```python
from build123d import *

# Parameters (mm, degrees)
SKETCH1_W               = 35
SKETCH1_H               = 17
BOSS_EXTRUDE1_DEPTH     = 0.5
SKETCH2_W               = 4.5
SKETCH2_H               = 8
BOSS_EXTRUDE2_DEPTH     = 3
SKETCH3_W               = 10.6
SKETCH3_H               = 15.6
BOSS_EXTRUDE3_DEPTH     = 1.5
CUT_EXTRUDE1_DEPTH      = 20.685019685
CUT_EXTRUDE1_DEPTH_BACK = 20.685019685
SKETCH4_R               = 1.1


with BuildPart() as part:
    # Sketch1 → Boss-Extrude1 (new, symmetric)
    with BuildSketch(Plane(origin=(0, 0, 0), x_dir=(1, 0, 0), z_dir=(0, 1, 0))):
        Rectangle(SKETCH1_W, SKETCH1_H)
    extrude(amount=BOSS_EXTRUDE1_DEPTH, both=True)

    # Sketch2 → Boss-Extrude2 (add)
    with BuildSketch(Plane(origin=(0, 0.5, 0), x_dir=(1, 0, 0), z_dir=(0, 1, 0))):
        with Locations((-15.25, -2.8)):
            Rectangle(SKETCH2_W, SKETCH2_H)
    extrude(amount=BOSS_EXTRUDE2_DEPTH)

    # Sketch3 → Boss-Extrude3 (add)
    with BuildSketch(Plane(origin=(0, 0.5, 0), x_dir=(1, 0, 0), z_dir=(0, 1, 0))):
        with Locations((-0.2, 0.1)):
            Rectangle(SKETCH3_W, SKETCH3_H)
    extrude(amount=BOSS_EXTRUDE3_DEPTH)

    # Sketch4 → Cut-Extrude1 (cut, two sides: drawn at the far end of the back side and taken through both)
    with BuildSketch(Plane(origin=(0, 0.5, 0), x_dir=(1, 0, 0), z_dir=(0, 1, 0)).offset(-CUT_EXTRUDE1_DEPTH_BACK)):
        with Locations(Location((15, 6, 0), (0, 0, 270))):
            Circle(SKETCH4_R)
        with Locations(Location((15, -6, 0), (0, 0, 270))):
            Circle(SKETCH4_R)
        with Locations(Location((-15, 6, 0), (0, 0, 270))):
            Circle(SKETCH4_R)
    extrude(amount=CUT_EXTRUDE1_DEPTH + CUT_EXTRUDE1_DEPTH_BACK, mode=Mode.SUBTRACT)


solid = part.part
```
Geometry check sheet. Reference: the model listing, model coordinates, mm. A direction names the side the tool comes from. Coordinates: 2 decimals unless noted, no trailing zeros. Write each loop counter-clockwise with the first axis right and the second up, starting at its lowest first coordinate (ties: lowest second). Pieces come first, ordered by that corner, then holes. Notation, with made-up numbers: (-26.75, -32) -> (17.25, -32) arc R27 cw to (17.25, 7) -> close; hole circle Ø11 at (82.25, 67.25). An arc over 180 degrees is marked (long way). Use CSV: the item, a comma, the result in double quotes. Start each with the question number.
Item 1: Cross-section at B-B, the plane z = 6. Record the cut outline in (x, y), plus the area to 3 significant figures.
Item 2: Cross-section at C-C, the plane x = -15. Record the cut outline in (y, z).
Item 3: Thickness scan on line 1 (X direction, y = -0.15, z = -6); line 2 (Z direction, x = 15, y = 0); line 3 (Z direction, x = -15, y = 0.1). Record the ranges inside material, lowest first.
Item 4: Mould release check, pull along Z, two halves, no side actions. Record for faces 4 (the flat face through (-15, 3.5, 3)), 5 (the cylindrical face through (13.926, -0.007, 5.762)), 6 (the flat face through (0, 1, 7.7)), 7 (the cylindrical face through (-16.074, -0.007, -6.238)): released by +Z, released by -Z, zero draft, split by the parting line, or undercut.
Item 5: Depth check by flat-ended pin: pin 1 Ø0.8 at (y, z) = (1.5, -1.5) entering from +X; pin 2 Ø1.3 at (x, z) = (-15, -6) entering from +Y (1 decimal); pin 3 Ø3 at (x, z) = (15, -6) entering from -Y; pin 4 Ø1.6 at (x, y) = (1.5, 1.5) entering from +Z. Enter the tip coordinate at first touch or a pass-through.
Item 6: Cross-section at A-A, the plane x = 15. Record the cut outline in (y, z), plus the area to 3 significant figures.
Item 7: Cross-section at D-D, the plane y = 1.6. Record the cut outline in (x, z), plus the area to 3 significant figures.
Item 8: Set-up check for faces 1 (the flat face through (-13, 2, 3)), 2 (the flat face through (5.1, 1, 0)), 3 (the flat face through (-15, 2, 6.8)): record each of +Z, -Z, +X, -X, +Y, -Y from which the full face is reachable in a straight line by a thin tool's end or side.
Answers:
1,outline,"(-17.5, -0.5) -> (13.9, -0.5) -> (13.9, 0.5) -> (5.1, 0.5) -> (5.1, 2) -> (-5.5, 2) -> (-5.5, 0.5) -> (-13, 0.5) -> (-13, 3.5) -> (-17.5, 3.5) -> close; (16.1, -0.5) -> (17.5, -0.5) -> (17.5, 0.5) -> (16.1, 0.5) -> close"
1,area,"62.2 mm^2"
2,outline,"(-0.5, -8.5) -> (0.5, -8.5) -> (0.5, -7.1) -> (-0.5, -7.1) -> close; (-0.5, -4.9) -> (0.5, -4.9) -> (0.5, -1.2) -> (3.5, -1.2) -> (3.5, 6.8) -> (0.5, 6.8) -> (0.5, 8.5) -> (-0.5, 8.5) -> close"
3,line 1,"-17.5 to -16.1, -13.9 to 13.9, 16.1 to 17.5"
3,line 2,"-8.5 to -7.1, -4.9 to 4.9, 7.1 to 8.5"
3,line 3,"-8.5 to -7.1, -4.9 to 8.5"
4,face 4,"zero draft"
4,face 5,"undercut"
4,face 6,"released by +Z"
4,face 7,"undercut"
5,pin 1,"x = 5.1"
5,pin 2,"through"
5,pin 3,"y = -0.5"
5,pin 4,"z = 7.7"
6,outline,"(-0.5, -8.5) -> (0.5, -8.5) -> (0.5, -7.1) -> (-0.5, -7.1) -> close; (-0.5, -4.9) -> (0.5, -4.9) -> (0.5, 4.9) -> (-0.5, 4.9) -> close; (-0.5, 7.1) -> (0.5, 7.1) -> (0.5, 8.5) -> (-0.5, 8.5) -> close"
6,area,"12.6 mm^2"
7,outline,"(-17.5, -1.2) -> (-13, -1.2) -> (-13, 6.8) -> (-17.5, 6.8) -> close; (-5.5, -7.9) -> (5.1, -7.9) -> (5.1, 7.7) -> (-5.5, 7.7) -> close"
7,area,"201 mm^2"
8,face 1,"+Z, -Z, +Y"
8,face 2,"+Z, -Z, +X, +Y"
8,face 3,"+Z, -X, +Y"
